from build123d import *

# Parameters (mm, degrees)
SKETCH1_R           = 2.54
BOSS_EXTRUDE1_DEPTH = 5.08
SKETCH2_R           = 5.08
SKETCH2_R_2         = 2.54
BOSS_EXTRUDE2_DEPTH = 1.27
SKETCH3_W           = 1.905
SKETCH3_H           = 3.81
BOSS_EXTRUDE3_DEPTH = 3.81
CUT_EXTRUDE1_REACH  = 10.799
SKETCH4_R           = 1.27


with BuildPart() as part:
    # Sketch1 → Boss-Extrude1 (new body)
    with BuildSketch(Plane(origin=(0, 0, 0), x_dir=(1, 0, 0), z_dir=(0, 1, 0))):
        with Locations(Location((0, 0, 0), (0, 0, 270))):
            Circle(SKETCH1_R)
    extrude(amount=BOSS_EXTRUDE1_DEPTH)

    # Sketch2 → Boss-Extrude2 (add)
    with BuildSketch(Plane.XZ):
        with Locations(Location((0, 0, 0), (0, 0, 270))):
            Circle(SKETCH2_R)
        with Locations(Location((0, 0, 0), (0, 0, 270))):
            Circle(SKETCH2_R_2, mode=Mode.SUBTRACT)
    extrude(amount=-BOSS_EXTRUDE2_DEPTH)

    # Sketch3 → Boss-Extrude3 (add)
    with BuildSketch(Plane.XZ):
        with Locations((0.9525, 0)):
            Rectangle(SKETCH3_W, SKETCH3_H)
    extrude(amount=BOSS_EXTRUDE3_DEPTH)

    # Sketch4 → Cut-Extrude1 (cut, up to next)
    with BuildSketch(Plane.ZY, mode=Mode.PRIVATE) as cut_extrude1_sk1:
        with Locations((0, -1.905)):
            Circle(SKETCH4_R)
    cut_extrude1_tool1 = extrude(cut_extrude1_sk1.sketch, amount=-CUT_EXTRUDE1_REACH, mode=Mode.PRIVATE) & part.part
    add(cut_extrude1_tool1.solids().sort_by_distance((0, -1.905, 0))[0], mode=Mode.SUBTRACT)


solid = part.part
Input: part model. Units: mm. Frame: model coordinates. A direction names the side the tool comes from. Coordinates: 2 decimals unless noted, no trailing zeros. Write each loop counter-clockwise with the first axis right and the second up, starting at its lowest first coordinate (ties: lowest second). Pieces come first, ordered by that corner, then holes. Notation, with made-up numbers: M 24.5,50.5 L 55.5,50.5 A24 cw 55.5,81.5 Z; hole C -18,45 d1. An arc over 180 degrees is marked long. Answer as a JSON object with one key per item and string values. Group by question number.
(1) Mould query, pull axis Z, two halves, no side actions, for faces 4 (the face through (5.037, 0.626, 0.661)), 5 (the face through (1, -2, 1.905)), 6 (the face through (0.94, -1.52, 1.21)), 7 (the face through (-1, 0, 0)). Classes: pulls with the +Z half, pulls with the -Z half, needs draft (parallel to the pull), parting line crosses it, or undercut.
(2) Section C-C on x = 1. Output: boundary loops of the cut face in (y, z) (3 decimals).
(3) Section A-A on y = -3. Output: boundary loops of the cut face in (x, z) (3 decimals), plus the area to 3 significant figures.
(4) Contact query for flat-ended pins moving along their axis: P1, Ø1.9, axis at y = -1.5, z = 0, coming from the +X side (3 decimals); P2, Ø1.5, axis at y = -0.5, z = -1.5, coming from the -X side; P3, Ø1.5, axis at x = -1, z = 0.5, coming from the -Y side. Output: stop coordinate, or through.
(5) Set-up query: faces 1 (the face through (-2, 1.27, -2)), 2 (the face through (1, -2, -1.905)), 3 (the face through (1, -3.81, 0)). Return all of +Z, -Z, +X, -X, +Y, -Y with unobstructed straight access to the full face (end or side cutting, diameter ignored); none if empty.
(6) Ray query, line 1 along Y through (x, z) = (1.1, 0) (3 decimals); line 2 along X through (y, z) = (-2, 1.5) (3 decimals); line 3 along Y through (x, z) = (-3.25, 0.75). Return the intervals inside material, ascending. Write a range as [from, to].
(7) Section D-D on y = 3.5. Output: boundary loops of the cut face in (x, z).
(8) Section B-B on z = 0. Output: boundary loops of the cut face in (x, y) (3 decimals).
Result set:
{
 "1": {"face 4": "parting line crosses it", "face 5": "pulls with the +Z half", "face 6": "undercut", "face 7": "needs draft"},
 "2": {"outline": "M -3.81,-1.905 L 0,-1.905 L 0,-4.981 L 1.27,-4.981 L 1.27,-2.335 L 5.08,-2.335 L 5.08,2.335 L 1.27,2.335 L 1.27,4.981 L 0,4.981 L 0,1.905 L -3.81,1.905 Z; hole C -1.905,0 d2.54"},
 "3": {"outline": "M 0,-1.905 L 1.905,-1.905 L 1.905,-0.643 L 0,-0.643 Z; M 0,0.643 L 1.905,0.643 L 1.905,1.905 L 0,1.905 Z", "area": "4.81 mm2"},
 "4": {"P1": "stops at x = 1.905", "P2": "stops at x = -4.99", "P3": "stops at y = 0"},
 "5": {"face 1": "+Y", "face 2": "-Z, +X, -X, -Y", "face 3": "+Z, -Z, +X, -X, -Y"},
 "6": {"line 1": "y = [-3.81, -3.175], [-0.635, 5.08]", "line 2": "x = [0, 1.905]", "line 3": "y = [0, 1.27]"},
 "7": {"outline": "C 0,0 d5.08"},
 "8": {"outline": "M -5.08,0 L 0,0 L 0,-0.635 L 1.905,-0.635 L 1.905,0 L 5.08,0 L 5.08,1.27 L 2.54,1.27 L 2.54,5.08 L -2.54,5.08 L -2.54,1.27 L -5.08,1.27 Z; M 0,-3.81 L 1.905,-3.81 L 1.905,-3.175 L 0,-3.175 Z"}
}
